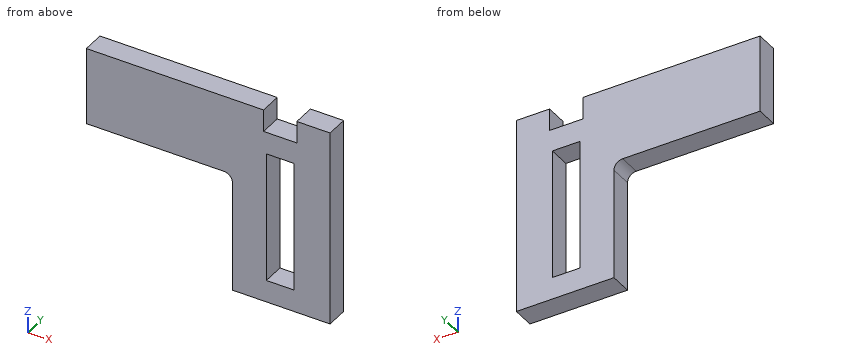
```python
from build123d import *

# Parameters (mm, degrees)
SKETCH1_W           = 31.742721484
SKETCH1_H           = 149.86
BOSS_EXTRUDE1_DEPTH = 25.4


with BuildPart() as part:
    # Sketch1 → Boss-Extrude1 (new body)
    with BuildSketch(Plane(origin=(0, 0, 0), x_dir=(1, 0, 0), z_dir=(0, 1, 0))):
        with BuildLine():
            Line((0, 0), (0, 88.9))
            Line((0, 88.9), (157.48, 88.9))
            ThreePointArc((157.48, 88.9), (164.551067812, 91.828932188), (167.48, 98.9))
            Line((167.48, 98.9), (167.48, 226.06))
            Line((167.48, 226.06), (279.4, 226.06))
            Line((279.4, 226.06), (279.4, 0))
            Line((279.4, 0), (241.3, 0))
            Line((241.3, 0), (241.3, 25.4))
            Line((241.3, 25.4), (203.2, 25.4))
            Line((203.2, 25.4), (203.2, 0))
            Line((203.2, 0), (0, 0))
        make_face()
        with Locations((222.25, 125.73)):
            Rectangle(SKETCH1_W, SKETCH1_H, mode=Mode.SUBTRACT)
    extrude(amount=BOSS_EXTRUDE1_DEPTH)


solid = part.part
```
Read the model definition and answer for the solid it produces. Units are mm, in the model's axes. Coordinates: 2 decimals unless noted, no trailing zeros. Loops run counter-clockwise (first coordinate to the right, second up) from the corner with the lowest first, then second, coordinate; pieces in that order, holes last. Notation, with made-up numbers: (53, 75) - (81, 75) arc R18 ccw to (81, 93) - close; hole circle Ø5 at (29, -17.5). An arc over 180 degrees is marked (long way). Answer in a Markdown table with one row per item.
1. Find section D-D, the plane x = 141. Write down the section's boundary in (y, z), then the cut area to 3 significant figures.
Conclusion:
| item | result |
|---|---|
| outline | (0, -88.9) - (25.4, -88.9) - (25.4, 0) - (0, 0) - close |
| area | 2,260 mm² |
2. Find section A-A, the plane z = -197. Write down the section's boundary in (x, y), then the cut area to 3 significant figures.
Conclusion:
| item | result |
|---|---|
| outline | (167.48, 0) - (206.38, 0) - (206.38, 25.4) - (167.48, 25.4) - close; (238.12, 0) - (279.4, 0) - (279.4, 25.4) - (238.12, 25.4) - close |
| area | 2,040 mm² |
3. Find section B-B, the plane y = 11.5. Write down the section's boundary in (x, z), then the cut area to 3 significant figures.
Conclusion:
| item | result |
|---|---|
| outline | (0, -88.9) - (157.48, -88.9) arc R10 cw to (167.48, -98.9) - (167.48, -226.06) - (279.4, -226.06) - (279.4, 0) - (241.3, 0) - (241.3, -25.4) - (203.2, -25.4) - (203.2, 0) - (0, 0) - close; hole (206.38, -200.66) - (238.12, -200.66) - (238.12, -50.8) - (206.38, -50.8) - close |
| area | 34,500 mm² |
4. Find section C-C, the plane x = 221. Write down the section's boundary in (y, z).
Conclusion:
| item | result |
|---|---|
| outline | (0, -226.06) - (25.4, -226.06) - (25.4, -200.66) - (0, -200.66) - close; (0, -50.8) - (25.4, -50.8) - (25.4, -25.4) - (0, -25.4) - close |
5. Given pin 1 (5 mm diameter, centred on x = 115, y = 17, fed in from -Z); pin 2 (12.5 mm diameter, centred on x = 230, y = 15, fed in from +Z); pin 3 (4 mm diameter, centred on x = 159.5, y = 7.5, fed in from -Z), each flat-ended and moving along its own axis, determine where each tip first touches the part or whether it passes through.
Conclusion:
| item | result |
|---|---|
| pin 1 | stops at z = -88.9 |
| pin 2 | stops at z = -25.4 |
| pin 3 | stops at z = -89.74 |
6. Straight lines are drawn through the part: line 1 (X direction, y = 2.5, z = -147); line 2 (X direction, y = 15.75, z = -66.5); line 3 (Z direction, x = 207, y = 11). For each, find the intervals that lie inside material, in ascending order.
Conclusion:
| item | result |
|---|---|
| line 1 | x = 167.48 to 206.38, 238.12 to 279.4 |
| line 2 | x = 0 to 206.38, 238.12 to 279.4 |
| line 3 | z = -226.06 to -200.66, -50.8 to -25.4 |
